```python
from build123d import *

# Parameters (mm, degrees)
EXTRUDE_1_DEPTH      = 2.2
EXTRUDE_2_DEPTH      = 3.25
SKETCH_3_W           = 50
SKETCH_3_H           = 10.05
EXTRUDE_3_DEPTH      = 3.25
CUT_EXTRUDE_1_DEPTH  = 30
EXTRUDE_4_REACH      = 56.389
SKETCH_6_R           = 5.025
SKETCH_8_R           = 1.675
SKETCH_8_R_2         = 0.84
CUT_EXTRUDE_3_DEPTH  = 55
SKETCH_9_W           = 28.473000816
SKETCH_9_H           = 14.532409192
CUT_EXTRUDE_4_DEPTH  = 3
EXTRUDE_5_DEPTH      = 2.45
SKETCH_11_W          = 12.614203935
SKETCH_11_H          = 10.05
EXTRUDE_6_DEPTH      = 3
SKETCH_12_W          = 36.628466797
SKETCH_12_H          = 15.348537224
CUT_EXTRUDE_5_DEPTH  = 10
SKETCH_13_W          = 5.35
SKETCH_13_H          = 5.35
CUT_EXTRUDE_6_DEPTH  = 14
SKETCH_14_R          = 1.1
CUT_EXTRUDE_7_DEPTH  = 14
SKETCH_15_R          = 1.1
CUT_EXTRUDE_8_DEPTH  = 10
SKETCH_16_R          = 1.625
EXTRUDE_7_DEPTH      = 5.7
SKETCH_17_W          = 19.923143876
SKETCH_17_H          = 15.083058075
CUT_EXTRUDE_9_DEPTH  = 3
SKETCH_18_R          = 1.675
SKETCH_18_R_2        = 1.6
CUT_EXTRUDE_10_DEPTH = 6


with BuildPart() as part:
    # 草图1 → 凸台-拉伸1 (new body)
    with BuildSketch(Plane.XY):
        with BuildLine():
            Line((1.539836705, 12.851012384), (15.55297303, 14.251012384))
            ThreePointArc((15.55297303, 14.251012384), (17.193415997, 16.063512384), (15.55297303, 17.876012384))
            Line((15.55297303, 17.876012384), (1.500532553, 18.901012384))
            ThreePointArc((1.500532553, 18.901012384), (0.527100583, 19.384612538), (-0.54702697, 19.551012384))
            Line((-0.54702697, 19.551012384), (-0.54702697, 20.901012384))
            Line((-0.54702697, 20.901012384), (19.51277613, 20.901012384))
            Line((19.51277613, 20.901012384), (41.45297303, 20.901012384))
            Line((41.45297303, 20.901012384), (41.45297303, 10.851012384))
            Line((41.45297303, 10.851012384), (-0.54702697, 10.851012384))
            Line((-0.54702697, 10.851012384), (-0.54702697, 12.201012384))
            ThreePointArc((-0.54702697, 12.201012384), (0.54584768, 12.367273294), (1.539836705, 12.851012384))
        make_face()
    extrude(amount=EXTRUDE_1_DEPTH)

    # 草图2 → 凸台-拉伸2 (add)
    with BuildSketch(Plane(origin=(0, 0, 0), x_dir=(-1, 0, 0), z_dir=(0, 0, -1))):
        Polygon((-19.51277613, 10.851012384), (-49.45297303, 10.851012384), (-49.45297303, 20.901012384), (-19.51277613, 20.901012384), (0.54702697, 20.901012384), (0.54702697, 10.851012384), align=None)
    extrude(amount=EXTRUDE_2_DEPTH)

    # 草图3 → 凸台-拉伸3 (add)
    with BuildSketch(Plane.XY.offset(2.2)):
        with Locations((24.45297303, 15.876012384)):
            Rectangle(SKETCH_3_W, SKETCH_3_H)
    extrude(amount=EXTRUDE_3_DEPTH)

    # 草图4 → 切除-拉伸1 (cut, symmetric)
    with BuildSketch(Plane.XY):
        with BuildLine():
            Line((-0.54702697, 19.551012384), (-2.235397712, 16.616091152))
            Line((-2.235397712, 16.616091152), (-1.110896638, 12.310548833))
            Line((-1.110896638, 12.310548833), (-0.54702697, 12.201012384))
            ThreePointArc((-0.54702697, 12.201012384), (0.54584768, 12.367273294), (1.539836705, 12.851012384))
            ThreePointArc((1.539836705, 12.851012384), (2.773180655, 15.88415254), (1.500532553, 18.901012384))
            ThreePointArc((1.500532553, 18.901012384), (0.527100583, 19.384612538), (-0.54702697, 19.551012384))
        make_face()
    extrude(amount=CUT_EXTRUDE_1_DEPTH, both=True, mode=Mode.SUBTRACT)

    # 凸台-拉伸4: up to this face of the body (flat: up to its plane)
    extrude_4_end = Plane(part.part.faces().sort_by_distance((25.407741746, 15.876338503, 5.45))[0])
    # 草图6 → 凸台-拉伸4 (add, up to the picked face)
    with BuildSketch(Plane(origin=(0, 0, -3.25), x_dir=(-1, 0, 0), z_dir=(0, 0, -1)), mode=Mode.PRIVATE) as extrude_4_sk1:
        with Locations(Location((-49.45297303, 15.876012384, 0), (0, 0, 90))):
            Circle(SKETCH_6_R)
    extrude_4_tool1 = split(extrude(extrude_4_sk1.sketch, amount=-EXTRUDE_4_REACH, mode=Mode.PRIVATE), bisect_by=extrude_4_end, keep=Keep.BOTH, mode=Mode.PRIVATE)
    add(extrude_4_tool1.solids().sort_by(Axis((49.452973, 15.876012, -3.25), (0, 0, 1)))[0])

    # 草图8 → 切除-拉伸3 (cut)
    with BuildSketch(Plane(origin=(0, 0, -3.25), x_dir=(-1, 0, 0), z_dir=(0, 0, -1))):
        with Locations((-49.45297303, 15.876012384)):
            Circle(SKETCH_8_R)
        with Locations(Location((-7.95297303, 15.856360308, 0), (0, 0, 180))):
            Circle(SKETCH_8_R_2)
    extrude(amount=-CUT_EXTRUDE_3_DEPTH, mode=Mode.SUBTRACT)

    # 草图9 → 切除-拉伸4 (cut)
    with BuildSketch(Plane(origin=(0, 0, -3.25), x_dir=(-1, 0, 0), z_dir=(0, 0, -1))):
        with Locations((-42.648638606, 15.039406696)):
            Rectangle(SKETCH_9_W, SKETCH_9_H)
    extrude(amount=-CUT_EXTRUDE_4_DEPTH, mode=Mode.SUBTRACT)

    # 草图10 → 凸台-拉伸5 (add)
    with BuildSketch(Plane(origin=(0, 0, 2.2), x_dir=(-1, 0, 0), z_dir=(0, 0, -1))):
        with BuildLine():
            Line((-49.45297303, 20.901012384), (-38.466384114, 20.901012384))
            Line((-38.466384114, 20.901012384), (-38.466384114, 10.851012384))
            Line((-38.466384114, 10.851012384), (-49.45297303, 10.851012384))
            ThreePointArc((-49.45297303, 10.851012384), (-46.217908976, 15.876012384), (-49.45297303, 20.901012384))
        make_face()
    extrude(amount=EXTRUDE_5_DEPTH)

    # 草图11 → 凸台-拉伸6 (add)
    with BuildSketch(Plane(origin=(0, 0, -3.25), x_dir=(-1, 0, 0), z_dir=(0, 0, -1))):
        with Locations((-32.625453647, 15.876012384)):
            Rectangle(SKETCH_11_W, SKETCH_11_H)
    extrude(amount=-EXTRUDE_6_DEPTH)

    # 草图12 → 切除-拉伸5 (cut)
    with BuildSketch(Plane(origin=(0, 0, -3.25), x_dir=(-1, 0, 0), z_dir=(0, 0, -1))):
        with Locations((-5.618322216, 15.103365543)):
            Rectangle(SKETCH_12_W, SKETCH_12_H)
    extrude(amount=-CUT_EXTRUDE_5_DEPTH, mode=Mode.SUBTRACT)

    # 草图13 → 切除-拉伸6 (cut)
    with BuildSketch(Plane.ZY.offset(-23.932555614)):
        with Locations((1.1, 16.124405573)):
            Rectangle(SKETCH_13_W, SKETCH_13_H)
    extrude(amount=-CUT_EXTRUDE_6_DEPTH, mode=Mode.SUBTRACT)

    # 草图14 → 切除-拉伸7 (cut)
    with BuildSketch(Plane(origin=(0, 20.901012384, 0), x_dir=(1, 0, 0), z_dir=(0, 1, 0))):
        with Locations(Location((30.538219594, -1.1, 0), (0, 0, 270))):
            Circle(SKETCH_14_R)
    extrude(amount=-CUT_EXTRUDE_7_DEPTH, mode=Mode.SUBTRACT)

    # 草图15 → 切除-拉伸8 (cut)
    with BuildSketch(Plane.XY.offset(5.45)):
        with Locations((36.879929969, 15.882801083)):
            Circle(SKETCH_15_R)
    extrude(amount=-CUT_EXTRUDE_8_DEPTH, mode=Mode.SUBTRACT)

    # 草图16 → 凸台-拉伸7 (add)
    with BuildSketch(Plane(origin=(0, 0, -0.25), x_dir=(-1, 0, 0), z_dir=(0, 0, -1))):
        with BuildLine():
            Line((-49.45297303, 20.901012384), (23.54702697, 20.901012384))
            ThreePointArc((23.54702697, 20.901012384), (28.57202697, 15.876012384), (23.54702697, 10.851012384))
            Line((23.54702697, 10.851012384), (-49.45297303, 10.851012384))
            Line((-49.45297303, 10.851012384), (-49.45297303, 20.901012384))
        make_face()
        with Locations((23.54702697, 15.876012384)):
            Circle(SKETCH_16_R, mode=Mode.SUBTRACT)
    extrude(amount=-EXTRUDE_7_DEPTH)

    # 草图17 → 切除-拉伸9 (cut)
    with BuildSketch(Plane(origin=(0, 0, -3.25), x_dir=(-1, 0, 0), z_dir=(0, 0, -1))):
        with Locations((-33.178239607, 16.007261263)):
            Rectangle(SKETCH_17_W, SKETCH_17_H)
    extrude(amount=-CUT_EXTRUDE_9_DEPTH, mode=Mode.SUBTRACT)

    # 草图18 → 切除-拉伸10 (cut)
    with BuildSketch(Plane(origin=(0, 0, -0.25), x_dir=(-1, 0, 0), z_dir=(0, 0, -1))):
        with Locations(Location((-49.45297303, 15.876012384, 0), (0, 0, 180))):
            Circle(SKETCH_18_R)
        with Locations((14.84318256, 15.876012384)):
            Circle(SKETCH_18_R_2)
        with BuildLine():
            Line((-31.661597205, 17.476012384), (8.461046927, 17.476012384))
            ThreePointArc((8.461046927, 17.476012384), (10.061046927, 15.876012384), (8.461046927, 14.276012384))
            Line((8.461046927, 14.276012384), (-31.661597205, 14.276012384))
            ThreePointArc((-31.661597205, 14.276012384), (-33.261597205, 15.876012384), (-31.661597205, 17.476012384))
        make_face()
    extrude(amount=-CUT_EXTRUDE_10_DEPTH, mode=Mode.SUBTRACT)


solid = part.part
```
Source: CAD feature listing. Evaluate the final solid. Frame: model axes, mm. A direction names the side the tool comes from. Coordinates: 2 decimals unless noted, no trailing zeros. Write each loop counter-clockwise with the first axis right and the second up, starting at its lowest first coordinate (ties: lowest second). Pieces come first, ordered by that corner, then holes. Notation, with made-up numbers: (28.25, 18.5) -> (78.25, 18.5) arc R10 cw to (78.25, 37.5) -> close; hole circle Ø9 at (61, 7). An arc over 180 degrees is marked (long way). Return JSON: item names as keys, results as strings. Group by question number.
1) Section query B-B, the plane z = 3.4. Return loops of the section in (x, y) (3 decimals), plus the area to 3 significant figures.
2) Section query C-C, the plane y = 13.25. Return loops of the section in (x, z).
3) Set-up query: faces 1 (the face through (13, 10.851, 3)), 2 (the face through (11, 14.276, 3)). Return all of +Z, -Z, +X, -X, +Y, -Y with unobstructed straight access to the full face (end or side cutting, diameter ignored); none if empty.
4) Mould query, pull axis X, two halves, no side actions, for faces 3 (the face through (-28.57, 15.99, 2.56)), 4 (the face through (14, 14, -0.25)), 5 (the face through (-15.581, 14.457, 2.56)). Classes: +X half, -X half, draft (parallel to the pull), parting line (faces both ways), or undercut.
5) Section query A-A, the plane x = 5. Return loops of the section in (y, z), plus the area to 3 significant figures.
6) Ray query, line 1 along X through (y, z) = (16, 0.35); line 2 along Y through (x, z) = (-7, 0.8); line 3 along X through (y, z) = (14.5, 2.1). Return the intervals inside material, ascending.
From the geometry:
{
 "1": {"outline": "(-23.547, 10.851) -> (49.453, 10.851) arc R5.025 ccw to (49.453, 20.901) -> (-23.547, 20.901) arc R5.025 ccw to start; hole circle Ø3.25 at (-23.547, 15.876); hole circle Ø3.2 at (-14.843, 15.876); hole (-8.461, 14.276) -> (31.662, 14.276) arc R1.6 ccw to (31.662, 17.476) -> (-8.461, 17.476) arc R1.6 ccw to start; hole circle Ø3.35 at (49.453, 15.876)", "area": "651 mm²"},
 "2": {"outline": "(-27.83, -0.25) -> (53.74, -0.25) -> (53.74, 5.45) -> (-27.83, 5.45) -> close"},
 "3": {"face 1": "+Z, -Z, +X, -X, -Y", "face 2": "+Z, -Z"},
 "4": {"face 3": "-X half", "face 4": "draft", "face 5": "undercut"},
 "5": {"outline": "(10.85, -0.25) -> (14.28, -0.25) -> (14.28, 5.45) -> (10.85, 5.45) -> close; (17.48, -0.25) -> (20.9, -0.25) -> (20.9, 5.45) -> (17.48, 5.45) -> close", "area": "39.0 mm²"},
 "6": {"line 1": "-28.57 to -25.17, -21.93 to -16.44, -13.25 to -10.06, 33.26 to 47.78, 51.12 to 54.48", "line 2": "10.85 to 14.28, 17.48 to 20.9", "line 3": "-28.38 to -24.41, -22.68 to -15.66, -14.03 to -9.28, 32.48 to 48.5, 50.41 to 54.29"}
}
